from build123d import *

# Parameters (mm, degrees)
ESQUISSE1_R                  = 4.5
BOSS_EXTRU_1_DEPTH           = 3
BOSS_EXTRU_2_START           = -0.5
ESQUISSE2_R                  = 0.75
BOSS_EXTRU_2_DEPTH           = 2
R_P_TITION_CIRCULAIRE1_COUNT = 2
ESQUISSE3_R                  = 0.75
BOSS_EXTRU_3_DEPTH           = 2
R_P_TITION_CIRCULAIRE2_COUNT = 2
ESQUISSE5_R                  = 4.5
ESQUISSE5_R_2                = 1.4
BOSS_EXTRU_4_DEPTH           = 0.7
ESQUISSE6_R                  = 4.5
ESQUISSE6_R_2                = 3
BOSS_EXTRU_5_DEPTH           = 0.8
ESQUISSE7_R                  = 3.75
ESQUISSE7_R_2                = 3
BOSS_EXTRU_6_DEPTH           = 0.8


with BuildPart() as part:
    # Esquisse1 → Boss.-Extru.1 (new body)
    with BuildSketch(Plane.XY):
        Circle(ESQUISSE1_R)
        Polygon((2.011577371, -1.550856692), (2.011577371, -2.011577371), (1.550856692, -2.011577371), (1.541643286, -2.018647066), (1.4224, -2.463669069), (0.977377998, -2.344425783), (0.966648759, -2.348869979), (0.73628842, -2.747865791), (0.337292608, -2.517505451), (0.325778716, -2.519021284), (0, -2.8448), (-0.325778716, -2.519021284), (-0.337292608, -2.517505451), (-0.73628842, -2.747865791), (-0.966648759, -2.348869979), (-0.977377998, -2.344425783), (-1.4224, -2.463669069), (-1.541643286, -2.018647066), (-1.550856692, -2.011577371), (-2.011577371, -2.011577371), (-2.011577371, -1.550856692), (-2.018647066, -1.541643286), (-2.463669069, -1.4224), (-2.344425783, -0.977377998), (-2.348869979, -0.966648759), (-2.747865791, -0.73628842), (-2.517505451, -0.337292608), (-2.519021284, -0.325778716), (-2.8448, 0), (-2.519021284, 0.325778716), (-2.517505451, 0.337292608), (-2.747865791, 0.73628842), (-2.348869979, 0.966648759), (-2.344425783, 0.977377998), (-2.463669069, 1.4224), (-2.018647066, 1.541643286), (-2.011577371, 1.550856692), (-2.011577371, 2.011577371), (-1.550856692, 2.011577371), (-1.541643286, 2.018647066), (-1.4224, 2.463669069), (-0.977377998, 2.344425783), (-0.966648759, 2.348869979), (-0.73628842, 2.747865791), (-0.337292608, 2.517505451), (-0.325778716, 2.519021284), (0, 2.8448), (0.325778716, 2.519021284), (0.337292608, 2.517505451), (0.73628842, 2.747865791), (0.966648759, 2.348869979), (0.977377998, 2.344425783), (1.4224, 2.463669069), (1.541643286, 2.018647066), (1.550856692, 2.011577371), (2.011577371, 2.011577371), (2.011577371, 1.550856692), (2.018647066, 1.541643286), (2.463669069, 1.4224), (2.344425783, 0.977377998), (2.348869979, 0.966648759), (2.747865791, 0.73628842), (2.517505451, 0.337292608), (2.519021284, 0.325778716), (2.8448, 0), (2.519021284, -0.325778716), (2.517505451, -0.337292608), (2.747865791, -0.73628842), (2.348869979, -0.966648759), (2.344425783, -0.977377998), (2.463669069, -1.4224), (2.018647066, -1.541643286), align=None, mode=Mode.SUBTRACT)
    extrude(amount=BOSS_EXTRU_1_DEPTH)

    # Esquisse2 → Boss.-Extru.2 (add)
    with BuildSketch(Plane.XY.offset(3).offset(BOSS_EXTRU_2_START)):
        with BuildLine():
            Line((-12.9, 2.467792536), (-0.72, 4.442026565))
            ThreePointArc((-0.72, 4.442026565), (-4.5, 0), (-0.72, -4.442026565))
            Line((-0.72, -4.442026565), (-12.9, -2.467792536))
            ThreePointArc((-12.9, -2.467792536), (-15, 0), (-12.9, 2.467792536))
        make_face()
        with Locations((-12.5, 0)):
            Circle(ESQUISSE2_R, mode=Mode.SUBTRACT)
        with Locations((-10, 0)):
            Circle(ESQUISSE2_R, mode=Mode.SUBTRACT)
        with Locations((-7.5, 0)):
            Circle(ESQUISSE2_R, mode=Mode.SUBTRACT)
    boss_extru_2 = extrude(amount=BOSS_EXTRU_2_DEPTH)

    # Répétition circulaire1: Boss.-Extru.2 ×2 about axis
    r_p_tition_circulaire1_axis = Axis((0, 0, 0), (0, 0, 1))
    for i in range(1, R_P_TITION_CIRCULAIRE1_COUNT):
        add(boss_extru_2.rotate(r_p_tition_circulaire1_axis, i * 360 / R_P_TITION_CIRCULAIRE1_COUNT))

    # Esquisse3 → Boss.-Extru.3 (add)
    with BuildSketch(Plane.XY.offset(4.5)):
        with BuildLine():
            Line((4.446426662, -0.692307692), (2.470237034, -13.384615385))
            ThreePointArc((2.470237034, -13.384615385), (0, -15.5), (-2.470237034, -13.384615385))
            Line((-2.470237034, -13.384615385), (-4.446426662, -0.692307692))
            ThreePointArc((-4.446426662, -0.692307692), (0, -4.5), (4.446426662, -0.692307692))
        make_face()
        with Locations((0, -13)):
            Circle(ESQUISSE3_R, mode=Mode.SUBTRACT)
        with Locations((0, -10.5)):
            Circle(ESQUISSE3_R, mode=Mode.SUBTRACT)
        with Locations((0, -8)):
            Circle(ESQUISSE3_R, mode=Mode.SUBTRACT)
    boss_extru_3 = extrude(amount=-BOSS_EXTRU_3_DEPTH)

    # Répétition circulaire2: Boss.-Extru.3 ×2 about axis
    r_p_tition_circulaire2_axis = Axis((0, 0, 0), (0, 0, 1))
    for i in range(1, R_P_TITION_CIRCULAIRE2_COUNT):
        add(boss_extru_3.rotate(r_p_tition_circulaire2_axis, i * 360 / R_P_TITION_CIRCULAIRE2_COUNT))

    # Esquisse5 → Boss.-Extru.4 (add)
    with BuildSketch(Plane.XY.offset(3)):
        Circle(ESQUISSE5_R)
        Circle(ESQUISSE5_R_2, mode=Mode.SUBTRACT)
    extrude(amount=BOSS_EXTRU_4_DEPTH)

    # Esquisse6 → Boss.-Extru.5 (add)
    with BuildSketch(Plane.XY.offset(3.7)):
        Circle(ESQUISSE6_R)
        Circle(ESQUISSE6_R_2, mode=Mode.SUBTRACT)
    extrude(amount=BOSS_EXTRU_5_DEPTH)

    # Esquisse7 → Boss.-Extru.6 (add)
    with BuildSketch(Plane.XY.offset(4.5)):
        Circle(ESQUISSE7_R)
        Circle(ESQUISSE7_R_2, mode=Mode.SUBTRACT)
    extrude(amount=BOSS_EXTRU_6_DEPTH)


solid = part.part
Read the model definition and answer for the solid it produces. Units are mm, in the model's axes. A direction names the side the tool comes from. Round coordinates to 2 decimals unless told otherwise and drop trailing zeros. Loops run counter-clockwise (first coordinate to the right, second up) from the corner with the lowest first, then second, coordinate; pieces in that order, holes last. Notation, with made-up numbers: (80.25, 46.25) - (138.25, 46.25) arc R23 ccw to (138.25, 59.25) - close; hole circle Ø6 at (11, 71.25). An arc over 180 degrees is marked (long way). One line per question, with ' | ' between items. Start each with the question number.
Q1. Section B-B on x = -7.5 is taken. Give the vertices of the cut face in (y, z).
Q2. For a pull along X with two mould halves and no side action, classify faces 1 (the flat face through (-8.485, 3.183, 3.486)), 2 (the cylindrical face through (0, 15.5, 3.5)), 3 (the cylindrical face through (-1.4, 0.06, 3.35)) as +X half, -X half, draft (parallel to the pull), parting line (faces both ways), or undercut.
Q3. For faces 4 (the cylindrical face through (-0.098, -12.256, 3.514)), 5 (the flat face through (-5, 0, 2.5)), 6 (the cylindrical face through (-3, 0, 4)), determine the directions among +Z, -Z, +X, -X, +Y, -Y from which every point of the face is accessible in a straight line to the end or side of a thin tool.
Q4. Section A-A on y = 8 is taken. Give the vertices of the cut face in (x, z), plus the area to 3 significant figures.
Q5. Flat-ended cylindrical pins translate along their axes: pin 1 (2 mm diameter, centred on x = 12.5, y = 0, fed in from -Z); pin 2 (1.4 mm diameter, centred on x = 10, y = 0, fed in from -Z); pin 3 (1.7 mm diameter, centred on x = 0, y = 13, fed in from +Z); pin 4 (3 mm diameter, centred on x = 11, z = 1.5, fed in from -Y). Find the tip coordinate at first contact, or state that the pin passes through.
Q6. Section C-C on x = 11.25 is taken. Give the vertices of the cut face in (y, z).
Q7. Find the intervals of material crossed by L1, parallel to Z at x = -7, y = -2; L2, parallel to Y at x = 12.5, z = 4.05; L3, parallel to X at y = 2, z = 4.1, in increasing order.
Established:
1) outline: (-3.34, 2.5) - (-0.75, 2.5) - (-0.75, 4.5) - (-3.34, 4.5) - close; (0.75, 2.5) - (3.34, 2.5) - (3.34, 4.5) - (0.75, 4.5) - close
2) face 1: -X half | face 2: parting line | face 3: undercut
3) face 4: +Z, -Z | face 5: -Z | face 6: +Z
4) outline: (-3.31, 2.5) - (-0.75, 2.5) - (-0.75, 4.5) - (-3.31, 4.5) - close; (0.75, 2.5) - (3.31, 2.5) - (3.31, 4.5) - (0.75, 4.5) - close | area: 10.2 mm²
5) pin 1: z = 2.5 | pin 2: through | pin 3: z = 4.5 | pin 4: y = -2.96
6) outline: (-2.74, 2.5) - (2.74, 2.5) - (2.74, 4.5) - (-2.74, 4.5) - close
7) L1: 2.5 to 4.5 | L2: -2.53 to -0.75, 0.75 to 2.53 | L3: -14 to -2.24, 2.24 to 14
